```python
from build123d import *

# Parameters (mm, degrees)
SKETCH1_W           = 680
SKETCH1_H           = 400
BOSS_EXTRUDE1_DEPTH = 20
SKETCH2_W           = 30
SKETCH2_H           = 27
CUT_EXTRUDE1_DEPTH  = 12
SKETCH3_R           = 3
CUT_EXTRUDE2_DEPTH  = 13
SKETCH4_R           = 3
CUT_EXTRUDE3_DEPTH  = 13


with BuildPart() as part:
    # Sketch1 → Boss-Extrude1 (new body)
    with BuildSketch(Plane(origin=(0, 0, 0), x_dir=(1, 0, 0), z_dir=(0, 1, 0))):
        Rectangle(SKETCH1_W, SKETCH1_H)
    extrude(amount=BOSS_EXTRUDE1_DEPTH)

    # Sketch2 → Cut-Extrude1 (cut)
    with BuildSketch(Plane(origin=(0, 20, 0), x_dir=(1, 0, 0), z_dir=(0, 1, 0))):
        with Locations((-305, -186.5)):
            Rectangle(SKETCH2_W, SKETCH2_H)
    cut_extrude1 = extrude(amount=-CUT_EXTRUDE1_DEPTH, mode=Mode.SUBTRACT)

    # Mirror1: Cut-Extrude1 across plane
    add(cut_extrude1.mirror(Plane.XY), mode=Mode.SUBTRACT)

    # Sketch3 → Cut-Extrude2 (cut)
    with BuildSketch(Plane(origin=(0, 20, 0), x_dir=(1, 0, 0), z_dir=(0, 1, 0))):
        with Locations(Location((321, -174, 0), (0, 0, 270))):
            Circle(SKETCH3_R)
        with Locations(Location((321, -142.5, 0), (0, 0, 270))):
            Circle(SKETCH3_R)
        with Locations(Location((321, -111, 0), (0, 0, 270))):
            Circle(SKETCH3_R)
    cut_extrude2 = extrude(amount=-CUT_EXTRUDE2_DEPTH, mode=Mode.SUBTRACT)

    # Mirror2: Cut-Extrude2 across plane
    add(cut_extrude2.mirror(Plane.XY), mode=Mode.SUBTRACT)

    # Sketch4 → Cut-Extrude3 (cut)
    with BuildSketch(Plane(origin=(0, 20, 0), x_dir=(1, 0, 0), z_dir=(0, 1, 0))):
        with Locations(Location((-325, -185, 0), (0, 0, 270))):
            Circle(SKETCH4_R)
        with Locations(Location((-285, -185, 0), (0, 0, 270))):
            Circle(SKETCH4_R)
    cut_extrude3 = extrude(amount=-CUT_EXTRUDE3_DEPTH, mode=Mode.SUBTRACT)

    # Mirror3: Cut-Extrude3 across plane
    add(cut_extrude3.mirror(Plane.XY), mode=Mode.SUBTRACT)


solid = part.part
```
Read the model definition and answer for the solid it produces. Units are mm, in the model's axes. A direction names the side the tool comes from. Coordinates: 2 decimals unless noted, no trailing zeros. Return JSON: item names as keys, results as strings.
1. A tool of negligible diameter and unlimited length cuts with its end or side. For faces 4 (the face through (-290, 14, -187)), 5 (the face through (-305, 8, 186)), 6 (the face through (-5, 0, -3)), from which of +Z, -Z, +X, -X, +Y, -Y can it reach the whole face along a straight path? Write none if from no direction.
Found:
{"face 4": "-Z, +Y", "face 5": "+Z, +Y", "face 6": "+Z, -Z, +X, -X, -Y"}
2. Each of these flat-tipped pins is pushed along its axis until it touches: P1, Ø3.5, axis at x = -285, z = -185, coming from the +Y side; P2, Ø9.5, axis at x = -308.5, y = 14.5, coming from the -Z side. Where does it stop, or does it pass through?
Found:
{"P1": "y = 7", "P2": "z = -173"}
3. Determine the mould class of faces 1 (the face through (-290, 14, 187)), 2 (the face through (-5, 20, -3)), 3 (the face through (-340, 10, 3)) for opening direction X: pulls with the +X half, pulls with the -X half, needs draft (parallel to the pull), parting line crosses it, or undercut.
Found:
{"face 1": "undercut", "face 2": "needs draft", "face 3": "pulls with the -X half"}
4. Find the intervals of material crossed by line 1 along X through (y, z) = (16.75, 185); line 2 along X through (y, z) = (13.5, 174); line 3 along X through (y, z) = (17.5, 178), in increasing order. Write a range as from..to.
Found:
{"line 1": "-340..-328, -322..-320, -290..-288, -282..340", "line 2": "-340..-320, -290..318, 324..340", "line 3": "-340..-320, -290..340"}
